The listing builds one solid part. Answer for the finished solid, in the listing's coordinates (mm). A direction names the side the tool comes from. Round coordinates to 2 decimals unless told otherwise and drop trailing zeros. Loops run counter-clockwise (first coordinate to the right, second up) from the corner with the lowest first, then second, coordinate; pieces in that order, holes last. Notation, with made-up numbers: (43, 89) -> (63, 89) arc R31 ccw to (63, 124) -> close; hole circle Ø11 at (78.5, -0.75). An arc over 180 degrees is marked (long way). Answer in a Markdown table with one row per item. Add a question column.
```python
from build123d import *

# Parameters (mm, degrees)
PAD_DEPTH       = 60
POCKET_DEPTH    = 60
SKETCH002_R     = 8
POCKET001_DEPTH = 5


with BuildPart() as part:
    # Sketch → Pad (new body)
    with BuildSketch(Plane.XZ):
        Polygon((0, 13.137292), (-24.148146, 6.666816), (-41.825815, -11.010853), (-48.296291, -35.158999), (-41.825815, -59.307145), (-24.148146, -76.984814), (0, -83.45529), (24.148146, -76.984814), (41.825815, -59.307145), (48.296291, -35.158999), (41.825815, -11.010853), (24.148146, 6.666816), align=None)
    extrude(amount=PAD_DEPTH)

    # Sketch001 (on Face13 of Pad) → Pocket (cut)
    with BuildSketch(Plane(origin=(0, 0, 0), x_dir=(1, 0, 0), z_dir=(0, 1, 0))):
        Polygon((0.278927, 81.474836), (23.169698, 75.240498), (40.032056, 58.422596), (46.155051, 34.895188), (40.08724, 11.999467), (23.293364, -4.858682), (-0.357735, -11.169546), (-23.145897, -4.936066), (-40.001684, 11.830942), (-46.296318, 35.16935), (-39.990105, 58.513313), (-22.910018, 75.414133), align=None)
    extrude(amount=-POCKET_DEPTH, mode=Mode.SUBTRACT)

    # Sketch002 (on Face11 of Pocket) → Pocket001 (cut)
    with BuildSketch(Plane(origin=(-50.56648, 0, -50.56648), x_dir=(0.707107, 0, -0.707107), z_dir=(-0.707107, 0, -0.707107))):
        with Locations((24.861167, 47)):
            Circle(SKETCH002_R)
        with Locations((24.861167, 21)):
            Circle(SKETCH002_R)
    extrude(amount=-POCKET001_DEPTH, mode=Mode.SUBTRACT)


solid = part.part
```
Item 1: Section C-C, the plane x = -18 is taken. Write down the section's boundary in (y, z), and give its area (3 significant figures).
Item 2: The mould has two halves that part along Y. Classify faces 3 (the flat face through (33.111, -29.58, -2.296)), 4 (the cylindrical face through (-36.472, -52.407, -63.292)): +Y half, -Y half, draft (parallel to the pull), parting line (faces both ways), or undercut.
Item 3: Section A-A, the plane y = -7 is taken. Write down the section's boundary in (x, z).
Item 4: Flat-ended cylindrical pins translate along their axes: P1, Ø2, axis at x = 7.5, y = -25.5, coming from the -Z side; P2, Ø1, axis at y = -31, z = -10, coming from the +X side; P3, Ø2, axis at x = -24, y = -6.5, coming from the -Z side. Find the tip coordinate at first contact, or state that the pin passes through.
Item 5: Section D-D, the plane y = -27 is taken. Write down the section's boundary in (x, z).
Item 6: Section B-B, the plane z = -55 is taken. Write down the section's boundary in (x, y).
Item 7: For faces 1 (the flat face through (-31.456, -29.58, -3.33)), 2 (the flat face through (-11.905, -29.58, 9.947)), determine the directions among +Z, -Z, +X, -X, +Y, -Y from which every point of the face is accessible in a straight line to the end or side of a thin tool.
Item 8: Consider L1, parallel to Z at x = 33, y = -53; L2, parallel to Z at x = -21.5, y = -20; L3, parallel to X at y = -6, z = -37.5. Determine where each line is inside the solid, lowest interval first. Write a range as from..to.
Here are the results:
| question | item | result |
|---|---|---|
| 1 | outline | (-60, -78.63) -> (0, -78.63) -> (0, -76.7) -> (-60, -76.7) -> close; (-60, 6.34) -> (0, 6.34) -> (0, 8.31) -> (-60, 8.31) -> close |
| 1 | area | 234 mm² |
| 2 | face 3 | draft |
| 2 | face 4 | undercut |
| 3 | outline | (-48.3, -35.16) -> (-41.83, -59.31) -> (-24.15, -76.98) -> (0, -83.46) -> (24.15, -76.98) -> (41.83, -59.31) -> (48.3, -35.16) -> (41.83, -11.01) -> (24.15, 6.67) -> (0, 13.14) -> (-24.15, 6.67) -> (-41.83, -11.01) -> close; hole (-46.3, -35.17) -> (-39.99, -58.51) -> (-22.91, -75.41) -> (0.28, -81.47) -> (23.17, -75.24) -> (40.03, -58.42) -> (46.16, -34.9) -> (40.09, -12) -> (23.29, 4.86) -> (-0.36, 11.17) -> (-23.15, 4.94) -> (-40, -11.83) -> close |
| 4 | P1 | stops at z = -81.71 |
| 4 | P2 | stops at x = 41.31 |
| 4 | P3 | stops at z = -77.29 |
| 5 | outline | (-48.3, -35.16) -> (-41.83, -59.31) -> (-36.73, -64.4) -> (-35.39, -63.07) -> (-39.99, -58.51) -> (-46.3, -35.17) -> (-40, -11.83) -> (-23.15, 4.94) -> (-0.36, 11.17) -> (23.29, 4.86) -> (40.09, -12) -> (46.16, -34.9) -> (40.03, -58.42) -> (23.17, -75.24) -> (0.28, -81.47) -> (-22.91, -75.41) -> (-27.87, -70.51) -> (-29.25, -71.89) -> (-24.15, -76.98) -> (0, -83.46) -> (24.15, -76.98) -> (41.83, -59.31) -> (48.3, -35.16) -> (41.83, -11.01) -> (24.15, 6.67) -> (0, 13.14) -> (-24.15, 6.67) -> (-41.83, -11.01) -> close |
| 6 | outline | (-42.98, -60) -> (-40.94, -60) -> (-40.94, 0) -> (-42.98, 0) -> close; (40.92, -60) -> (42.98, -60) -> (42.98, 0) -> (40.92, 0) -> close |
| 7 | face 1 | +Y, -Y |
| 7 | face 2 | +Z, -X, +Y, -Y |
| 8 | L1 | z = -68.13..-65.44, -4.89..-2.19 |
| 8 | L2 | z = -77.69..-75.78, 5.39..7.38 |
| 8 | L3 | x = -47.67..-45.67, 45.48..47.67 |
